Here's how the part is built. I have some questions about the finished solid (model axes, mm). Face numbers are marked on the shaded views. A direction names the side the tool comes from. Give positions to 0.01 mm unless a question says otherwise; leave off trailing zeros. Loops run counter-clockwise (first coordinate to the right, second up) from the corner with the lowest first, then second, coordinate; pieces in that order, holes last.
Q1. If we section it at A-A (y = -60): Please give me the cut outline in (x, z), plus the area to 3 significant figures.
Q2. If we section it at C-C (x = 25.5): Please give me the cut outline in (y, z), plus the area to 3 significant figures.
Q3. For the marked faces 1, 2 and 3, which set-ups out of +Z, -Z, +X, -X, +Y, -Y let a thin tool reach every point of the face, with its end or its side?
Q4. Will these pins go through, and if not, where does the flat tip stop? P1, Ø5, axis at x = 28.5, z = 19, coming from the -Y side; P2, Ø19, axis at x = 23.5, y = -57, coming from the +Z side; P3, Ø12, axis at x = 13.5, z = -10.5, coming from the -Y side; P4, Ø8, axis at x = -40.5, z = -16.5, coming from the +Y side.
Q5. If we section it at D-D (z = 3.5): Please give me the cut outline in (x, y), plus the area to 3 significant figures.
Q6. If we section it at B-B (z = -41): Please give me the cut outline in (x, y).
Q7. I need wall thicknesses on line 1 (X direction, y = -52, z = 1); line 2 (X direction, y = -131, z = -27.5); line 3 (Y direction, x = -59, z = -36.5). Which ranges of each line are inside material? Lowest first, please.
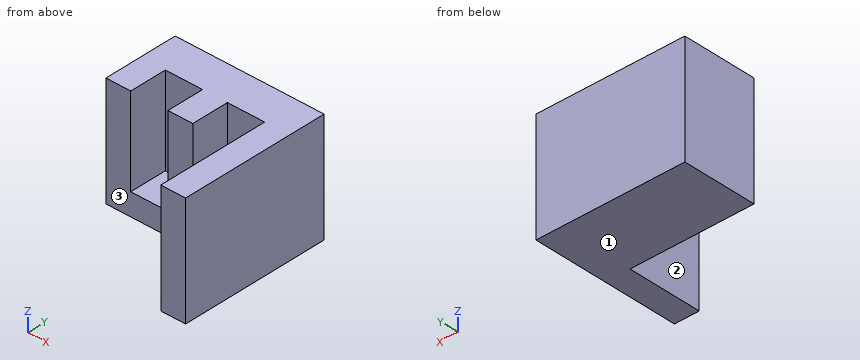
from build123d import *

# Parameters (mm, degrees)
F0_W     = 152.4
F0_H     = 114.3
F1_DEPTH = 152.4
F2_W     = 127
F2_H     = 114.3
F3_DEPTH = 76.2
F4_W     = 38.1
F4_H     = 91.44
F5_DEPTH = 38.1
F6_DEPTH = 38.1


with BuildPart() as f1:
    # F0 (on Front) → F1 (new body)
    with BuildSketch(Plane.XZ):
        Rectangle(F0_W, F0_H)
    extrude(amount=F1_DEPTH)

    # F2 (on face) → F3 (cut)
    with BuildSketch(Plane.XZ.offset(152.4)):
        with Locations((-12.7, 0)):
            Rectangle(F2_W, F2_H)
    extrude(amount=-F3_DEPTH, mode=Mode.SUBTRACT)

    # F4 (on face) → F5 (cut)
    with BuildSketch(Plane.XZ.offset(76.2)):
        with Locations((-31.75, 11.43)):
            Rectangle(F4_W, F4_H)
    extrude(amount=-F5_DEPTH, mode=Mode.SUBTRACT)

    # F4 (on face) → F6 (cut)
    with BuildSketch(Plane.XZ.offset(76.2)):
        with Locations((31.75, 11.43)):
            Rectangle(F4_W, F4_H)
    extrude(amount=-F6_DEPTH, mode=Mode.SUBTRACT)


solid = f1.part
Check sheet entries:
1. outline: (-76.2, -57.15) - (76.2, -57.15) - (76.2, 57.15) - (50.8, 57.15) - (50.8, -34.29) - (12.7, -34.29) - (12.7, 57.15) - (-12.7, 57.15) - (-12.7, -34.29) - (-50.8, -34.29) - (-50.8, 57.15) - (-76.2, 57.15) - close
1. area: 10,500 mm2
2. outline: (-76.2, -57.15) - (0, -57.15) - (0, 57.15) - (-38.1, 57.15) - (-38.1, -34.29) - (-76.2, -34.29) - close
2. area: 5,230 mm2
3. face 1: -Z, +X, -X, +Y, -Y
3. face 2: +Z, -Y
3. face 3: +Z, -Z, -X, -Y
4. P1: stops at y = -38.1
4. P2: stops at z = -34.29
4. P3: stops at y = -76.2
4. P4: stops at y = 0
5. outline: (-76.2, -76.2) - (-50.8, -76.2) - (-50.8, -38.1) - (-12.7, -38.1) - (-12.7, -76.2) - (12.7, -76.2) - (12.7, -38.1) - (50.8, -38.1) - (50.8, -152.4) - (76.2, -152.4) - (76.2, 0) - (-76.2, 0) - close
5. area: 10,600 mm2
6. outline: (-76.2, -76.2) - (50.8, -76.2) - (50.8, -152.4) - (76.2, -152.4) - (76.2, 0) - (-76.2, 0) - close
7. line 1: x = -76.2 to -50.8, -12.7 to 12.7, 50.8 to 76.2
7. line 2: x = 50.8 to 76.2
7. line 3: y = -76.2 to 0
